```python
from build123d import *

# Parameters (mm, degrees)
F0_R     = 7.5
F1_DEPTH = 3
F2_R     = 7.5
F3_DEPTH = 12
F4_SIZE2 = 3
F4_SIZE  = 12
F6_DEPTH = 4
F7_R     = 1.6
F8_DEPTH = 11


with BuildPart() as f1:
    # F0 (on Top) → F1 (new body)
    with BuildSketch(Plane.XY):
        with Locations((-11.8269938976, 14.5979337394)):
            Circle(F0_R)
    extrude(amount=F1_DEPTH)

    # F2 (on face) → F3 (join)
    with BuildSketch(Plane.XY.offset(3)):
        with Locations((-11.8269938976, 14.5979337394)):
            Circle(F2_R)
    extrude(amount=F3_DEPTH)

    # F4
    f4_edges = [f1.edges().sort_by_distance(p)[0] for p in [
        (-19.326994, 14.597934, 15),
    ]]
    f4_side = f1.faces().sort_by_distance((-19.326994, 14.597934, 7.5))[0]
    chamfer(f4_edges, length=F4_SIZE, length2=F4_SIZE2, reference=f4_side)

    # F5 (on face) → F6 (cut)
    with BuildSketch(Plane.XY.offset(15)):
        Polygon((-11.9095443248, 17.7979337394), (-14.6395504033, 16.1264429724), (-14.5569999761, 12.9264429724), (-11.7444434704, 11.3979337394), (-9.0144373918, 13.0694245065), (-9.096987819, 16.2694245065), align=None)
    extrude(amount=-F6_DEPTH, mode=Mode.SUBTRACT)

    # F7 (on face) → F8 (cut)
    with BuildSketch(Plane.XY.offset(11)):
        with Locations((-11.8269938976, 14.5979337394)):
            Circle(F7_R)
    extrude(amount=-F8_DEPTH, mode=Mode.SUBTRACT)


solid = f1.part
```
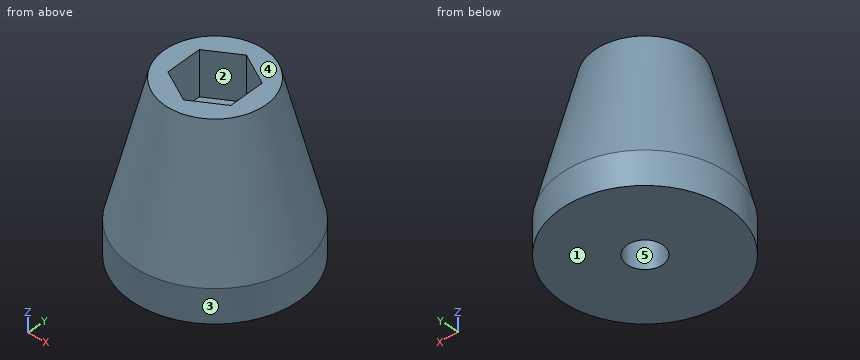
Part model, mm, in its own coordinate system. Face numbers are marked on the shaded views. A direction names the side the tool comes from. Round coordinates to 2 decimals unless told otherwise and drop trailing zeros. Loops run counter-clockwise (first coordinate to the right, second up) from the corner with the lowest first, then second, coordinate; pieces in that order, holes last.
1. Slice it at B-B (z = 3.75). Give the cut face in (x, y) (1 decimal), and give its area (3 significant figures).
Solutions:
outline: circle Ø14.6 at (-11.8, 14.6); hole circle Ø3.2 at (-11.8, 14.6)
area: 160 mm2
2. Drill centre lines: line 1 along X through (y, z) = (17.75, 14); line 2 along X through (y, z) = (16.75, 11.25); line 3 along Y through (x, z) = (-14.5, 12.25). Where is each one in solid material? Low to high.
Solutions:
line 1: x = -15.38 to -11.99, -11.82 to -8.27
line 2: x = -16.82 to -13.62, -9.98 to -6.83
line 3: y = 10.15 to 12.9, 16.21 to 19.04
3. Two-plate mould, pull along Y, no slides. Class the marked faces 3, 4 and 5: pulls with the +Y half, pulls with the -Y half, needs draft (parallel to the pull), parting line crosses it, or undercut.
Solutions:
face 3: parting line crosses it
face 4: needs draft
face 5: undercut
4. Slice it at A-A (z = 12.5). Give the cut face in (x, y) (3 decimals).
Solutions:
outline: circle Ø10.25 at (-11.827, 14.598); hole (-14.64, 16.126) - (-14.557, 12.926) - (-11.744, 11.398) - (-9.014, 13.069) - (-9.097, 16.269) - (-11.91, 17.798) - close
5. Flat gauge pins, fed straight in: pin 1 (5 mm diameter, centred on y = 15, z = 9, fed in from +X); pin 2 (5 mm diameter, centred on y = 20.5, z = 5.5, fed in from +X); pin 3 (6 mm diameter, centred on y = 16.5, z = 8, fed in from -X). Where does each tip first touch, or does it go through?
Solutions:
pin 1: stops at x = -5.21
pin 2: stops at x = -5.68
pin 3: stops at x = -18.73
6. 3-axis set-ups, long thin cutter, end or side, ignore diameter. For the marked faces 1 and 2: which of +Z, -Z, +X, -X, +Y, -Y reach the whole face in a straight line?
Solutions:
face 1: -Z, +X, -X, +Y, -Y
face 2: +Z
7. Slice it at C-C (z = 1.5). Give the cut face in (x, y).
Solutions:
outline: circle Ø15 at (-11.83, 14.6); hole circle Ø3.2 at (-11.83, 14.6)
